Could you check a few things on this model? Use its own coordinates, in mm. Face numbers are marked on the shaded views. Give positions to 0.01 mm unless a question says otherwise; leave off trailing zeros. Write each loop counter-clockwise with the first axis right and the second up, starting at its lowest first coordinate (ties: lowest second). Pieces come first, ordered by that corner, then holes. Notation, with made-up numbers: (-17.75, 2) - (-12.75, 2) arc R24 ccw to (-12.75, 26) - close; hole circle Ø5 at (11, -32). An arc over 180 degrees is marked (long way). Answer in a Markdown table with one row per item.
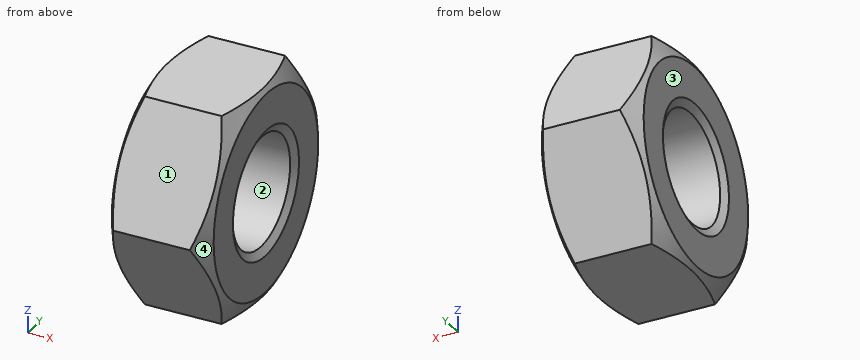
Autodesk Inventor part; units mm, degrees
ref_plane "Work Plane1" through (-56.8181, 0, 0) normal (0, -0.8660254, -0.5) x (1, 0, 0)
ref_plane "YZ Plane" through (0, 0, 0) normal (1, 0, 0) x (0, 1, 0)
ref_plane "XZ Plane" through (0, 0, 0) normal (0, 1, 0) x (-1, 0, 0)
sketch "Sketch1" plane through (0, 0, 0) normal (1, 0, 0) x (0, 1, 0)
  line L0 (-28.8675, 0) -> (-14.4338, 25)
  line L1 (-14.4338, 25) -> (14.4338, 25)
  line L2 (14.4338, 25) -> (28.8675, 0)
  line L3 (28.8675, 0) -> (14.4338, -25)
  line L4 (14.4338, -25) -> (-14.4338, -25)
  line L5 (-14.4338, -25) -> (-28.8675, 0)
  point P0 (0, 0)
  point P1 (0, 0)
  dimension "d0" = 57.735
extrude "Body" add sketch "Sketch1" along normal blind 24
sketch "Sketch2" plane through (0, 0, 0) normal (0, 0, 1) x (1, 0, 0)
  line L0 (0, 14.4338) -> (0, 28.8675)
  line L1 (0, 28.8675) -> (24, 28.8675)
  line L2 (24, 14.4338) -> (24, 28.8675)
  line L3 (-4.8, 0) -> (28.8, 0)
  line L4 (2.9546, 28.8675) -> (0, 23.75)
  line L5 (21.0454, 28.8675) -> (24, 23.75)
  dimension "d3" = 30
  dimension "d4" = 30
  dimension "d5" = 47.5
  dimension "d6" = 47.5
revolve "Chamfer1" cut sketch "Sketch2" angle 360 about axis through (-10, 0, 0) along (1, 0, 0)
sketch "Sketch3" plane through (24, 0, 0) normal (1, 0, 0) x (0, 0, -1)
  arc A0 (-0.625, -1.0825) -> (0.625, -1.0825) centre (0, 0) ccw
hole "Thread" at (24, 0, 0) direction (-1, 0, 0) diameter 26.211 end through all
chamfer "Chamfer2" distance 1.8944 angle 30 1 edges at (24, 0, 13.1055) measured on face at (24, 19.9399, -2.4211)
chamfer "Chamfer3" distance 1.8944 angle 30 1 edges at (0, 0, 13.1055) measured on face at (0, 19.9399, -2.4211)
ref_plane "Work Plane1" through (-56.8181, 0, 0) normal (0, -0.8660254, -0.5) x (1, 0, 0)
equation "\"d0\" = 1.1547 * SW"
equation "\"d1\" = KOH"
equation "\"d3\" = ANG1"
equation "\"d4\" = ANG2"
equation "\"d5\" = SW0"
equation "\"d6\" = SW01"
equation "\"d8\" = -0.5 * GD1 + 0.5 * NND"
equation "\"d40\" = -0.5 * GD1 + 0.5 * NND"
equation "\"d10\" = -0.5 * GD1 + 0.5 * NND"
equation "\"d41\" = -0.5 * GD1 + 0.5 * NND"
equation "\"ANG1\" = 30deg"
equation "\"ANG2\" = 30deg"
equation "\"KOH\" = 24"
equation "\"SW0\" = 47.5"
equation "\"SW01\" = SW0"
equation "\"GUL\" = 0.541266 * PTC"
equation "\"TOA\" = 30deg"
equation "\"PTC\" = 3.5"
equation "\"E0\" = 1.155 * SW"
equation "\"GAL\" = 0.541266 * PTC"
equation "\"Mw\" = 18.16"
properties part number "DIN 6915 - M30" material "Steel ASTM 194 2H"
1) We'd pull the mould along Y, two halves only. Please class the marked faces 1, 2, 3 and 4: +Y half, -Y half, draft (parallel to the pull), parting line (faces both ways), or undercut.
Check values:
| item | result |
|---|---|
| face 1 | -Y half |
| face 2 | undercut |
| face 3 | draft |
| face 4 | parting line |
2) Imagine slicing it at B-B (x = 15.5). List the corners of the cut face in (y, z) for me, then the cut area to 3 significant figures.
Check values:
| item | result |
|---|---|
| outline | (-28.87, 0) - (-14.43, -25) - (14.43, -25) - (28.87, 0) - (14.43, 25) - (-14.43, 25) - close; hole circle Ø26.21 at (0, 0) |
| area | 1,630 mm2 |
3) Will these pins go through, and if not, where does the flat tip stop? P1, Ø4, axis at x = 16, z = -7, coming from the +Y side; P2, Ø8, axis at x = 20.5, z = -16, coming from the -Y side; P3, Ø1.5, axis at y = 12.5, z = -11.5, coming from the -X side; P4, Ø6, axis at x = 6.5, y = -17.5, coming from the -Z side.
Check values:
| item | result |
|---|---|
| P1 | stops at y = 25.98 |
| P2 | stops at y = -21.94 |
| P3 | stops at x = 0 |
| P4 | stops at z = -24.89 |
4) If I drill on line 1 (Z direction, x = 10, y = 0); line 2 (Y direction, x = 17.25, z = 0); line 3 (Y direction, x = 6, z = 2), over which ranges is the centre line in solid material (lowest first)?
Check values:
| item | result |
|---|---|
| line 1 | z = -25 to -13.11, 13.11 to 25 |
| line 2 | y = -28.87 to -13.11, 13.11 to 28.87 |
| line 3 | y = -27.71 to -12.95, 12.95 to 27.71 |
5) Imagine slicing it at A-A (y = 0). List the corners of the cut face in (x, z) for me.
Check values:
| item | result |
|---|---|
| outline | (0, -23.75) - (0.72, -25) - (23.28, -25) - (24, -23.75) - (24, -15) - (22.91, -13.11) - (1.09, -13.11) - (0, -15) - close; (0, 15) - (1.09, 13.11) - (22.91, 13.11) - (24, 15) - (24, 23.75) - (23.28, 25) - (0.72, 25) - (0, 23.75) - close |
